from build123d import *

# Parameters (mm, degrees)
SKETCH2_R           = 1.7
BOSS_EXTRUDE2_DEPTH = 10


with BuildPart() as part:
    # Sketch2 → Boss-Extrude2 (new body)
    with BuildSketch(Plane(origin=(0, 0, 0), x_dir=(1, 0, 0), z_dir=(0, 1, 0))):
        Polygon((-44.162144835, 83.28125), (47.234241277, 83.28125), (47.234241277, 68.28125), (14.234241277, 68.28125), (-44.162144835, 68.28125), align=None)
        with Locations((-38.719051078, 78.587953022)):
            Circle(SKETCH2_R, mode=Mode.SUBTRACT)
        with Locations((22.234241277, 74.963265867)):
            Circle(SKETCH2_R, mode=Mode.SUBTRACT)
    extrude(amount=BOSS_EXTRUDE2_DEPTH)


solid = part.part
Source: CAD feature listing. Evaluate the final solid. Frame: model axes, mm. Round coordinates to 2 decimals unless told otherwise and drop trailing zeros.
Q1. Mould query, pull axis Z, two halves, no side actions, for faces 1 (the face through (1, 5, -83.281)), 2 (the face through (-40.417, 4.93, -78.663)), 3 (the face through (-44.162, 5, -76)). Classes: pulls with the +Z half, pulls with the -Z half, needs draft (parallel to the pull), parting line crosses it, or undercut.
Q2. Ray query, line 1 (X direction, y = 7.75, z = -74.25); line 2 (X direction, y = 4.25, z = -78.5). Return the intervals inside material, ascending.
Q3. First-contact query: P1, Ø2.5, axis at x = -38.72, z = -78.59, coming from the -Y side. Flat tip, straight axial feed; report the tip coordinate or a pass-through.
Solutions:
1. face 1: pulls with the -Z half
1. face 2: undercut
1. face 3: needs draft
2. line 1: x = -44.16 to 20.69, 23.78 to 47.23
2. line 2: x = -44.16 to -40.42, -37.02 to 47.23
3. P1: passes through
